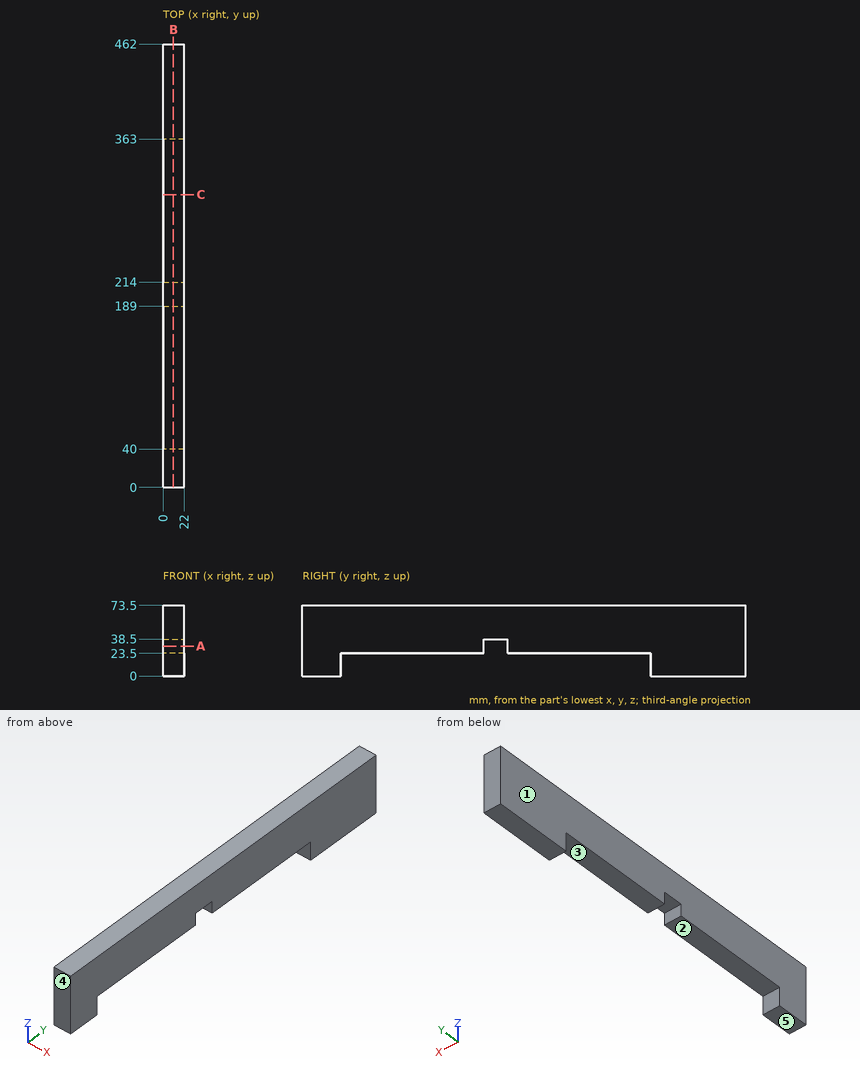
Study the drawing (mm; zero at the part's minimum x, y, z) and answer. A direction names the side the tool comes from. Give positions to 0.01 mm unless a question says otherwise; leave off trailing zeros. Order: outer loops, then holes, each group sorted by start corner. A loop starts at its lowest first (then second) coordinate and runs counter-clockwise, first axis right, second up.
1. Section B-B, the plane x = 10.5 is taken. Determine the outline of the cut face in (y, z).
Result sheet:
outline: (0, 0) - (40, 0) - (40, 23.5) - (189, 23.5) - (189, 38.5) - (214, 38.5) - (214, 23.5) - (363, 23.5) - (363, 0) - (462, 0) - (462, 73.5) - (0, 73.5) - close
2. Section C-C, the plane y = 305 is taken. Determine the outline of the cut face in (x, z).
Result sheet:
outline: (0, 23.5) - (22, 23.5) - (22, 73.5) - (0, 73.5) - close
3. Each of these flat-tipped pins is pushed along its axis until it touches: P1, Ø5, axis at x = 12.5, z = 35, coming from the -Y side; P2, Ø1.5, axis at x = 14.5, y = 56, coming from the -Z side; P3, Ø11, axis at x = 9, y = 198, coming from the -Z side. Where does it stop, or does it pass through?
Result sheet:
P1: stops at y = 0
P2: stops at z = 23.5
P3: stops at z = 38.5
4. The mould has two halves that part along Y. Classify the marked faces 3, 4 and 5: released by +Y, released by -Y, zero draft, split by the parting line, or undercut.
Result sheet:
face 3: undercut
face 4: released by -Y
face 5: zero draft
5. Straight lines are drawn through the part: L1, parallel to Z at x = 17.25, y = 224.5; L2, parallel to Y at x = 19, z = 14; L3, parallel to Y at x = 6.5, z = 33.5. For each, find the intervals that lie inside material, in ascending order.
Result sheet:
L1: z = 23.5 to 73.5
L2: y = 0 to 40, 363 to 462
L3: y = 0 to 189, 214 to 462
6. For the marked faces 1 and 2, determine the directions among +Z, -Z, +X, -X, +Y, -Y from which every point of the face is accessible in a straight line to the end or side of a thin tool.
Result sheet:
face 1: +Z, -Z, -X, +Y, -Y
face 2: -Z, +X, -X
7. Section A-A, the plane z = 31 is taken. Determine the outline of the cut face in (x, y), and give its area (3 significant figures).
Result sheet:
outline: (0, 0) - (22, 0) - (22, 189) - (0, 189) - close; (0, 214) - (22, 214) - (22, 462) - (0, 462) - close
area: 9,610 mm2
